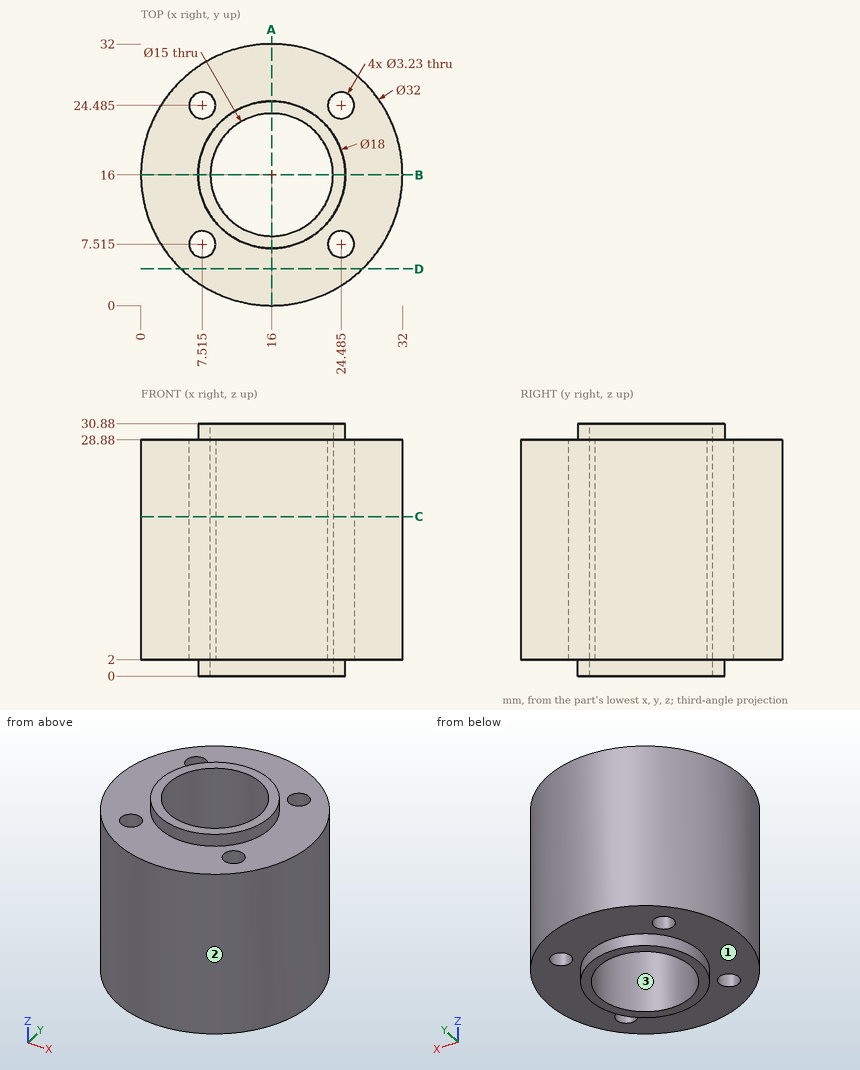
Here's the drawing with two shaded views (mm, measured from the low corner). I have some questions. Round coordinates to 2 decimals unless told otherwise and drop trailing zeros. Loops run counter-clockwise (first coordinate to the right, second up) from the corner with the lowest first, then second, coordinate; pieces in that order, holes last. Notation, with made-up numbers: (0.5, -10.5) - (16.5, -10.5) arc R34 cw to (16.5, 20.5) - close; hole circle Ø4 at (51.25, 38.5). An arc over 180 degrees is marked (long way). Use CSV: the item, a comma, the result in double quotes. Start each with the question number.
1) We'd pull the mould along Y, two halves only. Please class the marked faces 1, 2 and 3: released by +Y, released by -Y, zero draft, split by the parting line, or undercut.
2) If we section it at C-C on z = 19.5: Write out the boundary of the cut face in (x, y) (3 decimals), plus the area to 3 significant figures.
3) Please list where these lines run through material, in increasing order: probe 1 along Y at (x, z) = (25, 27.5); probe 2 along Y at (x, z) = (8, 7.5); probe 3 along Z at (x, y) = (5, 9). Write a range as [from, to].
4) If we section it at D-D on y = 4.5: Write out the boundary of the cut face in (x, z), plus the area to 3 significant figures.
5) If we section it at A-A on x = 16: Write out the boundary of the cut face in (y, z), plus the area to 3 significant figures.
6) For pin 1 Ø8 at (y, z) = (22.5, 6.5) entering from -X; pin 2 Ø3 at (x, y) = (11, 3.5) entering from -Z; pin 3 Ø3 at (x, z) = (7.5, 15) entering from +Y, each with a flat end and sliding along its axis, tell me the tip position at first contact or that it passes through.
Geometry results:
1,face 1,"zero draft"
1,face 2,"split by the parting line"
1,face 3,"undercut"
2,outline,"circle Ø32 at (16, 16); hole circle Ø3.23 at (7.515, 7.515); hole circle Ø3.23 at (7.515, 24.485); hole circle Ø15 at (16, 16); hole circle Ø3.23 at (24.485, 7.515); hole circle Ø3.23 at (24.485, 24.485)"
2,area,"595 mm2"
3,probe 1,"y = [2.77, 5.98], [9.05, 22.95], [26.02, 29.23]"
3,probe 2,"y = [2.14, 5.97], [9.06, 22.94], [26.03, 29.86]"
3,probe 3,"z = [2, 28.88]"
4,outline,"(4.88, 2) - (27.12, 2) - (27.12, 28.88) - (4.88, 28.88) - close"
4,area,"598 mm2"
5,outline,"(0, 2) - (7, 2) - (7, 0) - (8.5, 0) - (8.5, 30.88) - (7, 30.88) - (7, 28.88) - (0, 28.88) - close; (23.5, 0) - (25, 0) - (25, 2) - (32, 2) - (32, 28.88) - (25, 28.88) - (25, 30.88) - (23.5, 30.88) - close"
5,area,"469 mm2"
6,pin 1,"stops at x = 0.2"
6,pin 2,"stops at z = 2"
6,pin 3,"stops at y = 30.39"
